Verification items for the finished model (mm, model axes). Round coordinates to 2 decimals unless told otherwise and drop trailing zeros. Order: outer loops, then holes, each group sorted by start corner. A loop starts at its lowest first (then second) coordinate and runs counter-clockwise, first axis right, second up. Notation, with made-up numbers: (-39, -14) -> (-34, -14) arc R11 cw to (-34, 3) -> close; hole circle Ø11 at (-29.5, 24). An arc over 180 degrees is marked (long way). Return JSON: item names as keys, results as strings. Group by question number.
Item 1: Sectioned sample at B-B on x = -116.5. Record the cut outline in (y, z).
Item 2: Sectioned sample at A-A on z = 3.75. Record the cut outline in (x, y), plus the area to 3 significant figures.
Item 3: Scan lines: probe 1 along Y at (x, z) = (0, 4.5); probe 2 along Y at (x, z) = (-150, 0.5); probe 3 along Y at (x, z) = (175, 1.75). Record each from-to range of solid material in increasing order. Write a range as from..to.
Item 4: Depth check by flat-ended pin: pin 1 Ø8 at (x, y) = (0, 19) entering from +Z; pin 2 Ø2 at (x, z) = (119.5, 4) entering from -Y; pin 3 Ø0.9 at (y, z) = (19, 5.5) entering from +X; pin 4 Ø17 at (x, y) = (0, 19) entering from -Z. Enter the tip coordinate at first touch or a pass-through.
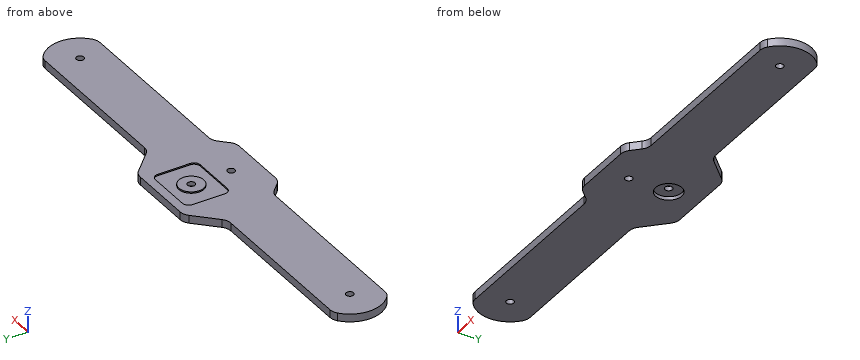
```python
from build123d import *

# Parameters (mm, degrees)
F0_R     = 3
F1_DEPTH = 6.35
F2_R     = 10
F3_R     = 10.5
F4_DEPTH = 2.75
F5_R     = 10
F6_DEPTH = 1.1


# Not quite as in the source:
# - a feature names something its author has since deleted; it is built from what else it names


with BuildPart() as f1:
    # F0 (on Top) → F1 (new body)
    with BuildSketch(Plane.XY):
        with BuildLine():
            Line((25.8578643763, 44), (0, 44))
            Line((0, 44), (-25.8578643763, 44))
            ThreePointArc((-25.8578643763, 44), (-29.6846986999, 43.2387953251), (-32.9289321881, 41.0710678119))
            Line((-32.9289321881, 41.0710678119), (-49.0710678119, 24.9289321881))
            ThreePointArc((-49.0710678119, 24.9289321881), (-52.3153013001, 22.7612046749), (-56.1421356237, 22))
            Line((-56.1421356237, 22), (-187.8528743982, 22))
            ThreePointArc((-187.8528743982, 22), (-200.4793324147, 0), (-187.8528743982, -22))
            Line((-187.8528743982, -22), (-43.6421356237, -22))
            ThreePointArc((-43.6421356237, -22), (-39.8153013001, -22.7612046749), (-36.5710678119, -24.9289321881))
            Line((-36.5710678119, -24.9289321881), (-30.4289321881, -31.0710678119))
            ThreePointArc((-30.4289321881, -31.0710678119), (-27.1846986999, -33.2387953251), (-23.3578643763, -34))
            Line((-23.3578643763, -34), (0, -34))
            Line((0, -34), (23.3578643763, -34))
            ThreePointArc((23.3578643763, -34), (27.1846986999, -33.2387953251), (30.4289321881, -31.0710678119))
            Line((30.4289321881, -31.0710678119), (36.5710678119, -24.9289321881))
            ThreePointArc((36.5710678119, -24.9289321881), (39.8153013001, -22.7612046749), (43.6421356237, -22))
            Line((43.6421356237, -22), (187.8528743982, -22))
            ThreePointArc((187.8528743982, -22), (200.4793324147, 0), (187.8528743982, 22))
            Line((187.8528743982, 22), (56.1421356237, 22))
            ThreePointArc((56.1421356237, 22), (52.3153013001, 22.7612046749), (49.0710678119, 24.9289321881))
            Line((49.0710678119, 24.9289321881), (32.9289321881, 41.0710678119))
            ThreePointArc((32.9289321881, 41.0710678119), (29.6846986999, 43.2387953251), (25.8578643763, 44))
        make_face()
        with Locations((-175, 0)):
            Circle(F0_R, mode=Mode.SUBTRACT)
        with Locations((0, -13)):
            Circle(F0_R, mode=Mode.SUBTRACT)
        with Locations((175, 0)):
            Circle(F0_R, mode=Mode.SUBTRACT)
        with Locations((0, 19)):
            Circle(F0_R, mode=Mode.SUBTRACT)
    extrude(amount=F1_DEPTH)

    # F2
    f2_edges = [f1.edges().sort_by_distance(p)[0] for p in [
        (-187.852874, 22, 3.175),
        (-187.852874, -22, 3.175),
        (187.852874, -22, 3.175),
        (187.852874, 22, 3.175),
    ]]
    fillet(f2_edges, radius=F2_R)

    # F3 (on face) → F4 (cut)
    with BuildSketch(Plane(origin=(0, 0, 0), x_dir=(1, 0, 0), z_dir=(0, 0, -1))):
        with Locations((0, -19)):
            Circle(F3_R)
    extrude(amount=-F4_DEPTH, mode=Mode.SUBTRACT)

    # F5 (on face) → F6 (cut)
    with BuildSketch(Plane.XY.offset(6.35)):
        with BuildLine():
            ThreePointArc((22.5, 32), (21.0355339059, 35.5355339059), (17.5, 37))
            Line((17.5, 37), (-17.5, 37))
            ThreePointArc((-17.5, 37), (-21.0355339059, 35.5355339059), (-22.5, 32))
            Line((-22.5, 32), (-22.5, 6))
            ThreePointArc((-22.5, 6), (-21.0355339059, 2.4644660941), (-17.5, 1))
            Line((-17.5, 1), (17.5, 1))
            ThreePointArc((17.5, 1), (21.0355339059, 2.4644660941), (22.5, 6))
            Line((22.5, 6), (22.5, 32))
        make_face()
        with Locations((0, 19)):
            Circle(F5_R, mode=Mode.SUBTRACT)
    extrude(amount=-F6_DEPTH, mode=Mode.SUBTRACT)


solid = f1.part
```
Recorded:
{
 "1": {"outline": "(-22, 0) -> (22, 0) -> (22, 6.35) -> (-22, 6.35) -> close"},
 "2": {"outline": "(-191.09, -19.75) arc R10 ccw to (-184.78, -22) -> (-43.64, -22) arc R10 cw to (-36.57, -24.93) -> (-30.43, -31.07) arc R10 ccw to (-23.36, -34) -> (23.36, -34) arc R10 ccw to (30.43, -31.07) -> (36.57, -24.93) arc R10 cw to (43.64, -22) -> (184.78, -22) arc R10 ccw to (191.09, -19.75) arc R25.48 ccw to (191.09, 19.75) arc R10 ccw to (184.78, 22) -> (56.14, 22) arc R10 cw to (49.07, 24.93) -> (32.93, 41.07) arc R10 ccw to (25.86, 44) -> (-25.86, 44) arc R10 ccw to (-32.93, 41.07) -> (-49.07, 24.93) arc R10 cw to (-56.14, 22) -> (-184.78, 22) arc R10 ccw to (-191.09, 19.75) arc R25.48 ccw to start; hole circle Ø6 at (-175, 0); hole circle Ø6 at (0, -13); hole circle Ø6 at (0, 19); hole circle Ø6 at (175, 0)", "area": "19,800 mm²"},
 "3": {"probe 1": "-34..-16, -10..16, 22..44", "probe 2": "-22..22", "probe 3": "-22..-3, 3..22"},
 "4": {"pin 1": "z = 6.35", "pin 2": "y = -22", "pin 3": "x = 192.47", "pin 4": "z = 2.75"}
}
